```python
from build123d import *

# Parameters (mm, degrees)
BOX003_W                 = 101.6
BOX003_H                 = 279.4
BOX003_DEPTH             = 12.7
BOX009_W                 = 12.7
BOX009_H                 = 44.1376
BOX009_DEPTH             = 139.7
BOX006_W                 = 12.7
BOX006_H                 = 44.1376
BOX006_DEPTH             = 139.7
BOX007_W                 = 12.7
BOX007_H                 = 44.1376
BOX007_DEPTH             = 139.7
SKETCH002_W              = 165.100117
SKETCH002_H              = 139.700117
SKETCH002_R              = 6.6548
SKETCH002_R_2            = 63.4873
PAD_DEPTH                = 12.7
CLONE001_PLACEMENT_ANGLE = 180
CLONE_PLACEMENT_ANGLE    = 180
BOX010_W                 = 165.1
BOX010_H                 = 12.7
BOX010_DEPTH             = 139.7
SKETCH004_R              = 63.4873
POCKET_DEPTH             = 12.7
BOX008_W                 = 12.7
BOX008_H                 = 44.1376
BOX008_DEPTH             = 139.7
BOX_W                    = 127
BOX_H                    = 114.3
BOX_DEPTH                = 139.7
BOX002_W                 = 12.7
BOX002_H                 = 279.4
BOX002_DEPTH             = 139.7
SKETCH003_R              = 12.7
SKETCH003_W              = 101.6
SKETCH003_H              = 101.6
POCKET003005_DEPTH       = 139.7


with BuildPart() as cube003:
    # Box003 → Box003 (new body)
    with BuildSketch(Plane(origin=(-224.636743, 494.971814, 58.555664), x_dir=(1, 0, 0), z_dir=(0, 0, 1))):
        with Locations((50.8, 139.7)):
            Rectangle(BOX003_W, BOX003_H)
    extrude(amount=BOX003_DEPTH)


with BuildPart() as cube009:
    # Box009 → Box009 (new body)
    with BuildSketch(Plane(origin=(-91.286743, 901.371814, -68.444336), x_dir=(1, 0, 0), z_dir=(0, 0, 1))):
        with Locations((6.35, 22.0688)):
            Rectangle(BOX009_W, BOX009_H)
    extrude(amount=BOX009_DEPTH)


with BuildPart() as cube006:
    # Box006 → Box006 (new body)
    with BuildSketch(Plane(origin=(-243.686743, 323.834214, -68.444336), x_dir=(1, 0, 0), z_dir=(0, 0, 1))):
        with Locations((6.35, 22.0688)):
            Rectangle(BOX006_W, BOX006_H)
    extrude(amount=BOX006_DEPTH)


with BuildPart() as cube007:
    # Box007 → Box007 (new body)
    with BuildSketch(Plane(origin=(-243.686743, 901.371814, -68.444336), x_dir=(1, 0, 0), z_dir=(0, 0, 1))):
        with Locations((6.35, 22.0688)):
            Rectangle(BOX007_W, BOX007_H)
    extrude(amount=BOX007_DEPTH)


with BuildPart() as pad:
    # Sketch002 → Pad (new body)
    with BuildSketch(Plane(origin=(0, 37.338, 0), x_dir=(-1, 0, 0), z_dir=(0, 1, 0))):
        with Locations((-69.215058, 89.86448)):
            Rectangle(SKETCH002_W, SKETCH002_H)
        with Locations((-121.408307, 142.057728)):
            Circle(SKETCH002_R, mode=Mode.SUBTRACT)
        with Locations((-17.02181, 142.057728)):
            Circle(SKETCH002_R, mode=Mode.SUBTRACT)
        with Locations((-17.02181, 37.671231)):
            Circle(SKETCH002_R, mode=Mode.SUBTRACT)
        with Locations((-121.408307, 37.671231)):
            Circle(SKETCH002_R, mode=Mode.SUBTRACT)
        with Locations((-69.215, 89.864421)):
            Circle(SKETCH002_R_2, mode=Mode.SUBTRACT)
    extrude(amount=PAD_DEPTH)


with BuildPart() as clone_of_pad001:
    # Clone001 base: copy of Pad
    add(pad.part)


with BuildPart() as clone_of_pad001_1:
    # Clone001 placement: moved
    add(clone_of_pad001.part.moved(Location((-91.921743, 995.547414, -88.458874))).rotate(Axis((-91.921743, 995.547414, -88.458874), (0, 0, 1)), CLONE001_PLACEMENT_ANGLE))


with BuildPart() as clone_of_pad:
    # Clone base: copy of Pad
    add(pad.part)


with BuildPart() as clone_of_pad_1:
    # Clone placement: moved
    add(clone_of_pad.part.moved(Location((-91.921626, 361.172214, -88.458874))).rotate(Axis((-91.921626, 361.172214, -88.458874), (0, 0, 1)), CLONE_PLACEMENT_ANGLE))


with BuildPart() as pocket:
    # Box010 → Box010 (new body)
    with BuildSketch(Plane(origin=(-102.435181, 88.203278, -436.376007), x_dir=(1, 0, 0), z_dir=(0, 0, 1))):
        with Locations((82.55, 6.35)):
            Rectangle(BOX010_W, BOX010_H)
    extrude(amount=BOX010_DEPTH)

    # Sketch004 → Pocket (cut)
    with BuildSketch(Plane(origin=(-102.435181, 88.203278, -436.376007), x_dir=(1, 0, 0), z_dir=(0, -1, 0))):
        with Locations((82.55, 69.85)):
            Circle(SKETCH004_R)
    extrude(amount=-POCKET_DEPTH, mode=Mode.SUBTRACT)


with BuildPart() as clone_of_pocket003005005:
    # Clone006 base: copy of Pocket
    add(pocket.part)


with BuildPart() as clone_of_pocket003005005_1:
    # Clone006 placement: moved
    add(clone_of_pocket003005005.part.moved(Location((-141.251562, 800.468536, 367.931671))))


with BuildPart() as clone_of_pocket:
    # Clone005 base: copy of Pocket
    add(pocket.part)


with BuildPart() as clone_of_pocket_1:
    # Clone005 placement: moved
    add(clone_of_pocket.part.moved(Location((-141.251562, 279.768536, 367.931671))))


with BuildPart() as cube008:
    # Box008 → Box008 (new body)
    with BuildSketch(Plane(origin=(-91.286743, 323.834214, -68.444336), x_dir=(1, 0, 0), z_dir=(0, 0, 1))):
        with Locations((6.35, 22.0688)):
            Rectangle(BOX008_W, BOX008_H)
    extrude(amount=BOX008_DEPTH)


with BuildPart() as cube:
    # Box → Box (new body)
    with BuildSketch(Plane(origin=(-224.636743, 380.671814, -68.444336), x_dir=(1, 0, 0), z_dir=(0, 0, 1))):
        with Locations((63.5, 57.15)):
            Rectangle(BOX_W, BOX_H)
    extrude(amount=BOX_DEPTH)


with BuildPart() as clone_of_cube:
    # Clone008 base: copy of Cube
    add(cube.part)


with BuildPart() as clone_of_cube_1:
    # Clone008 placement: moved
    add(clone_of_cube.part.moved(Location((0, 393.7, 0))))


with BuildPart() as pocket003005:
    # Box002 → Box002 (new body)
    with BuildSketch(Plane(origin=(-123.036743, 494.971814, -68.444336), x_dir=(1, 0, 0), z_dir=(0, 0, 1))):
        with Locations((6.35, 139.7)):
            Rectangle(BOX002_W, BOX002_H)
    extrude(amount=BOX002_DEPTH)

    # Fusion: union Cube003, Cube009, Cube006, Cube007, Clone of Pad001, Clone of Pad, Clone of Pocket003005005, Clone of Pocket, Cube008, Clone of Cube, Cube
    add(cube003.part)
    add(cube009.part)
    add(cube006.part)
    add(cube007.part)
    add(clone_of_pad001_1.part)
    add(clone_of_pad_1.part)
    add(clone_of_pocket003005005_1.part)
    add(clone_of_pocket_1.part)
    add(cube008.part)
    add(clone_of_cube_1.part)
    add(cube.part)


with BuildPart() as pocket003005_1:
    # Clone009 placement: moved
    add(pocket003005.part.moved(Location((-550.744446, 1129.268555, -180.039734))))

    # Sketch003 → Pocket003005 (cut)
    with BuildSketch(Plane(origin=(-550.744446, 1129.268555, -108.78407), x_dir=(1, 0, 0), z_dir=(0, 0, 1))):
        with Locations((-161.136743, 634.671814)):
            Circle(SKETCH003_R)
        with Locations((-161.136743, 837.871814)):
            Rectangle(SKETCH003_W, SKETCH003_H)
        with Locations((-161.136743, 431.471814)):
            Rectangle(SKETCH003_W, SKETCH003_H)
    extrude(amount=-POCKET003005_DEPTH, mode=Mode.SUBTRACT)


solid = pocket003005_1.part
```
Input: part model. Units: mm. Frame: model coordinates. A direction names the side the tool comes from. Round coordinates to 2 decimals unless told otherwise and drop trailing zeros. Loops run counter-clockwise (first coordinate to the right, second up) from the corner with the lowest first, then second, coordinate; pieces in that order, holes last. Notation, with made-up numbers: M 79,49 L 116,49 A28 cw 116,73 Z; hole C -35,30 d3. An arc over 180 degrees is marked long. Answer in a Markdown table with one row per item. Add a question column.
1. Contact query for flat-ended pins moving along their axis: pin 1 (2 mm diameter, centred on x = -721.5, z = -124.5, fed in from +Y); pin 2 (8 mm diameter, centred on x = -691, z = -228.5, fed in from -Y); pin 3 (2 mm diameter, centred on y = 1621.5, z = -164, fed in from +X). Output: stop coordinate, or through.
2. Section B-B (y = 1727). Output: boundary loops of the cut face in (x, z).
3. Mould query, pull axis Y, two halves, no side actions, for faces 1 (the face through (-768, 1440.403, -209)), 2 (the face through (-724.57, 1764.5, -115.05)), 3 (the face through (-794.431, 1447, -180)). Classes: released by +Y, released by -Y, zero draft, split by the parting line, or undercut.
4. Set-up query: faces 4 (the face through (-673.781, 1762, -186)), 5 (the face through (-661.081, 1762, -180)), 6 (the face through (-775.381, 1760, -118)), 7 (the face through (-653.54, 2081.22, -128.99)), 8 (the face through (-762.681, 1560, -178)). Return all of +Z, -Z, +X, -X, +Y, -Y with unobstructed straight access to the full face (end or side cutting, diameter ignored); none if empty.
5. Ray query, probe 1 along Y at (x, z) = (-672.5, -232.5); probe 2 along Y at (x, z) = (-653, -128); probe 3 along Y at (x, z) = (-745.5, -167.5). Return the intervals inside material, ascending.
6. Section A-A (y = 1565). Output: boundary loops of the cut face in (x, z).
Values follow:
| question | item | result |
|---|---|---|
| 1 | pin 1 | y = 1916.34 |
| 1 | pin 2 | y = 1611.54 |
| 1 | pin 3 | x = -648.38 |
| 2 | outline | M -775.38,-121.48 L -673.78,-121.48 L -673.78,-248.48 L -661.08,-248.48 L -661.08,-108.78 L -775.38,-108.78 Z |
| 3 | face 1 | released by -Y |
| 3 | face 2 | undercut |
| 3 | face 3 | zero draft |
| 4 | face 4 | -Z, -X |
| 4 | face 5 | +Z, -Z, +X |
| 4 | face 6 | +Z, -Z, -X |
| 4 | face 7 | +Y |
| 4 | face 8 | +Z, -Z |
| 5 | probe 1 | 1440.4 to 1453.1, 1497.24 to 1509.94, 1611.54 to 1916.34, 2017.94 to 2030.64, 2074.78 to 2087.48 |
| 5 | probe 2 | 1440.4 to 1453.1, 1497.24 to 1624.24, 1903.64 to 2030.64, 2074.78 to 2087.48 |
| 5 | probe 3 | 1611.54 to 1624.24, 1903.64 to 1916.34 |
| 6 | outline | M -775.38,-248.48 L -762.68,-248.48 L -762.68,-108.78 L -775.38,-108.78 Z; M -661.08,-248.48 L -648.38,-248.48 L -648.38,-108.78 L -661.08,-108.78 Z |
